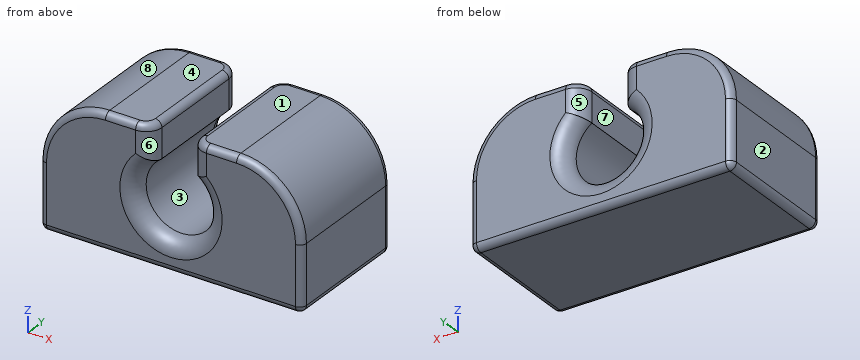
```python
from build123d import *

# Parameters (mm, degrees)
F2_DEPTH = 0.8
F3_DEPTH = 10
F4_R     = 1.2
F5_R     = 5
F6_R     = 0.5


# Not quite as in the source:
# - a feature names something its author has since deleted; it is built from what else it names


with BuildPart() as f2:
    # F1 (on Front) → F2 (new body)
    with BuildSketch(Plane.XZ):
        with BuildLine():
            Line((8.5, 20), (0, 20))
            Line((0, 20), (0, 10))
            Line((0, 10), (20, 10))
            Line((20, 10), (20, 20))
            Line((20, 20), (11.5, 20))
            Line((11.5, 20), (11.5, 17.2449944321))
            ThreePointArc((11.5, 17.2449944321), (10, 12.3), (8.5, 17.2449944321))
            Line((8.5, 17.2449944321), (8.5, 20))
        make_face()
    extrude(amount=F2_DEPTH)

    # F1 (on Front) → F3 (join)
    with BuildSketch(Plane.XZ):
        with BuildLine():
            Line((8.5, 20), (0, 20))
            Line((0, 20), (0, 10))
            Line((0, 10), (20, 10))
            Line((20, 10), (20, 20))
            Line((20, 20), (11.5, 20))
            Line((11.5, 20), (11.5, 17.2449944321))
            ThreePointArc((11.5, 17.2449944321), (10, 12.3), (8.5, 17.2449944321))
            Line((8.5, 17.2449944321), (8.5, 20))
        make_face()
    extrude(amount=F3_DEPTH)

    # F4
    f4_edges = [f2.edges().sort_by_distance(p)[0] for p in [
        (10, -10, 12.3),
        (8.5, -10, 18.622497),
        (11.5, -10, 18.622497),
        (10, 0, 12.3),
        (8.5, 0, 18.622497),
        (11.5, 0, 18.622497),
    ]]
    fillet(f4_edges, radius=F4_R)

    # F5
    f5_edges = [f2.edges().sort_by_distance(p)[0] for p in [
        (20, -5, 20),
        (0, -5, 20),
    ]]
    fillet(f5_edges, radius=F5_R)

    # F6
    f6_edges = [f2.edges().sort_by_distance(p)[0] for p in [
        (1.464466, -10, 18.535534),
        (0, -10, 12.5),
        (10, -10, 10),
        (18.535534, -10, 18.535534),
        (18.535534, 0, 18.535534),
        (1.464466, 0, 18.535534),
        (20, -5, 10),
        (0, -5, 10),
        (10, 0, 10),
    ]]
    fillet(f6_edges, radius=F6_R)


solid = f2.part
```
Here's how the part is built. I have some questions about the finished solid (model axes, mm). Face numbers are marked on the shaded views. A direction names the side the tool comes from. Coordinates: 2 decimals unless noted, no trailing zeros. Order: outer loops, then holes, each group sorted by start corner. A loop starts at its lowest first (then second) coordinate and runs counter-clockwise, first axis right, second up. Notation, with made-up numbers: (-15.5, 29) -> (20.5, 29) arc R27 ccw to (20.5, 60) -> close; hole circle Ø5 at (68, 23). An arc over 180 degrees is marked (long way). Return JSON: item names as keys, results as strings.
1) Thinking about a two-plate mould opening in X: for the marked faces 1, 2 and 3, which applies, +X half, -X half, draft (parallel to the pull), parting line (faces both ways), or undercut?
Conclusion:
{"face 1": "draft", "face 2": "-X half", "face 3": "undercut"}
2) If we section it at A-A on y = -5.25: List the corners of the cut face in (x, z) for me (3 decimals), plus the area to 3 significant figures.
Conclusion:
{"outline": "(0, 10.5) arc R0.5 ccw to (0.5, 10) -> (19.5, 10) arc R0.5 ccw to (20, 10.5) -> (20, 15) arc R5 ccw to (15, 20) -> (12, 20) arc R0.5 ccw to (11.5, 19.5) -> (11.5, 17.245) arc R2.7 cw (long way) to (8.5, 17.245) -> (8.5, 19.5) arc R0.5 ccw to (8, 20) -> (5, 20) arc R5 ccw to (0, 15) -> close", "area": "159 mm²"}
3) If I drill on probe 1 along X at (y, z) = (-8.25, 15); probe 2 along Z at (x, y) = (10, -5.5); probe 3 along X at (y, z) = (-1, 16), over which ranges is the centre line in solid material (lowest first)?
Conclusion:
{"probe 1": "x = 0 to 7.3, 12.7 to 20", "probe 2": "z = 10 to 12.3", "probe 3": "x = 0.1 to 7.47, 12.53 to 19.9"}
4) I'm going to push flat-ended pins straight in: P1, Ø2, axis at y = -2, z = 16, coming from the -X side; P2, Ø2.5, axis at y = -7, z = 18, coming from the +X side; P3, Ø1.1, axis at y = -4.5, z = 18.5, coming from the -X side. Where does each tip first touch, or does it pass through?
Conclusion:
{"P1": "stops at x = 0", "P2": "stops at x = 19.68", "P3": "stops at x = 0.96"}
5) If we section it at B-B on x = 10: List the corners of the cut face in (y, z) for me, plus the area to 3 significant figures.
Conclusion:
{"outline": "(-10, 10.5) arc R0.5 ccw to (-9.5, 10) -> (-0.5, 10) arc R0.5 ccw to (0, 10.5) -> (0, 11.1) arc R1.2 ccw to (-1.2, 12.3) -> (-8.8, 12.3) arc R1.2 ccw to (-10, 11.1) -> close", "area": "22.3 mm²"}
6) On a 3-axis mill with a long thin cutter (end or side, diameter ignored), from which of +Z, -Z, +X, -X, +Y, -Y can I reach the whole of each face in a straight line? I mean the marked faces 4, 5, 6, 7 and 8. Say none if no direction works.
Conclusion:
{"face 4": "+Z, +X, -X, +Y, -Y", "face 5": "+Z, +Y", "face 6": "+Z, -Y", "face 7": "+Z, +Y, -Y", "face 8": "+Z, -X, +Y, -Y"}
